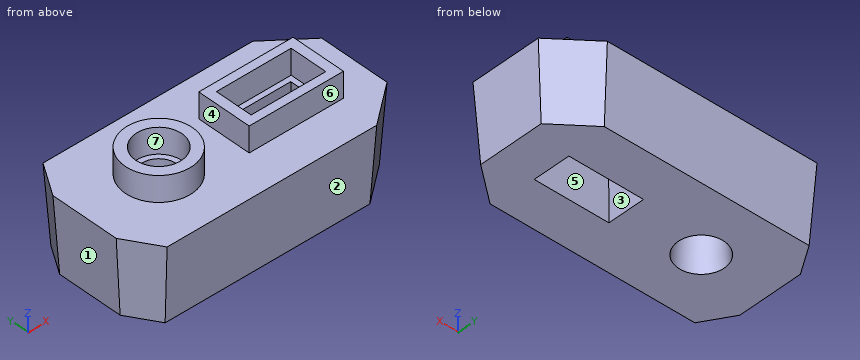
from build123d import *

# Parameters (mm, degrees)
SKETCH1_R           = 12.7
SKETCH1_W           = 41.2
SKETCH1_H           = 20.6
BOSS_EXTRUDE1_DEPTH = 42
BOSS_EXTRUDE1_DRAFT = -4
SKETCH2_R           = 18.5
SKETCH2_R_2         = 12.7
SKETCH2_W           = 52
SKETCH2_H           = 30
SKETCH2_W_2         = 41.2
SKETCH2_H_2         = 20.6
BOSS_EXTRUDE2_DEPTH = 56


with BuildPart() as part:
    # Sketch1 → Boss-Extrude1 (with draft: the straight prism first)
    with BuildSketch(Plane.XY):
        Polygon((-28, 34), (-38, 18), (-38, -18), (-28, -34), (85, -34), (105, -18), (105, 18), (85, 34), align=None)
        Circle(SKETCH1_R, mode=Mode.SUBTRACT)
        with Locations((62, 0)):
            Rectangle(SKETCH1_W, SKETCH1_H, mode=Mode.SUBTRACT)
    extrude(amount=BOSS_EXTRUDE1_DEPTH)
    # Boss-Extrude1: the draft: its side faces are tilted about the plane it starts from
    boss_extrude1_sides = [part.faces().sort_by_distance(p)[0] for p in [
        (-33, 26, 21),
        (-38, 0, 21),
        (-33, -26, 21),
        (28.5, -34, 21),
        (95, -26, 21),
        (105, 0, 21),
        (95, 26, 21),
        (28.5, 34, 21),
        (-12.7, 0, 21),
        (41.4, 0, 21),
        (62, 10.3, 21),
        (82.6, 0, 21),
        (62, -10.3, 21),
    ]]
    draft(boss_extrude1_sides, Plane.XY, BOSS_EXTRUDE1_DRAFT)

    # Sketch2 → Boss-Extrude2 (add)
    # profile 1 of 2: a face of its own
    with BuildSketch(Plane.XY):
        with Locations(Location((0, 0, 0), (0, 0, 180))):
            Circle(SKETCH2_R)
        with Locations(Location((0, 0, 0), (0, 0, 180))):
            Circle(SKETCH2_R_2, mode=Mode.SUBTRACT)
    # profile 2 of 2: a face of its own
    with BuildSketch(Plane.XY):
        with Locations((62, 0)):
            Rectangle(SKETCH2_W, SKETCH2_H)
        with Locations((62, 0)):
            Rectangle(SKETCH2_W_2, SKETCH2_H_2, mode=Mode.SUBTRACT)
    extrude(amount=BOSS_EXTRUDE2_DEPTH)


solid = part.part
Geometry: final body of the model. Coordinates: model frame, mm. Face numbers are marked on the shaded views. A direction names the side the tool comes from. Coordinates: 2 decimals unless noted, no trailing zeros. Loops run counter-clockwise (first coordinate to the right, second up) from the corner with the lowest first, then second, coordinate; pieces in that order, holes last. Notation, with made-up numbers: M 44,39 L 56,39 A18 cw 56,58 Z; hole C 18,-4 d11. An arc over 180 degrees is marked long. One line per item, written item: value. Start each with the question number.
1) Pin query (flat end, axial travel): P1, Ø4, axis at x = 74.5, z = 48.5, coming from the +Y side; P2, Ø16.5, axis at x = 60.5, y = -1.5, coming from the +Z side; P3, Ø7, axis at x = 58, z = 46, coming from the -Y side. Return the tip coordinate at first contact, or that it passes through.
2) Reachability of the marked faces 4, 5, 6 and 7 from +Z, -Z, +X, -X, +Y, -Y: full face, straight path, thin tool, end or side. Return the list, or none.
3) Cut plane A-A (z = 52). Return loops of the section in (x, y), then the cut area to 3 significant figures.
4) Cut plane B-B (x = 66). Return loops of the section in (y, z).
5) Draft query along Y for the marked faces 1, 2 and 3. Return one class per face: released by +Y, released by -Y, zero draft, split by the parting line, or undercut.
6) Cut plane C-C (y = 0). Return loops of the section in (x, z), then the cut area to 3 significant figures.
7) Cut plane D-D (z = 12). Return loops of the section in (x, y).
8) Material intervals for L1, parallel to Y at x = 0, z = 48.5; L2, parallel to Y at x = 52, z = 54; L3, parallel to X at y = -0.5, z = 28, sorted ascending. Write a range as from..to.
Evaluation:
1. P1: y = 15
1. P2: z = 42
1. P3: y = -15
2. face 4: +Z, +Y, -Y
2. face 5: -Z
2. face 6: +Z, +X, -Y
2. face 7: +Z
3. outline: C 0,0 d37; M 36,-15 L 88,-15 L 88,15 L 36,15 Z; hole C 0,0 d25.4; hole M 41.4,-10.3 L 82.6,-10.3 L 82.6,10.3 L 41.4,10.3 Z
3. area: 1,280 mm^2
4. outline: M -36.94,42 L -34,0 L -10.3,0 L -7.36,42 L -10.3,42 L -10.3,56 L -15,56 L -15,42 Z; M 7.36,42 L 10.3,0 L 34,0 L 36.94,42 L 15,42 L 15,56 L 10.3,56 L 10.3,42 Z
5. face 1: zero draft
5. face 2: released by -Y
5. face 3: undercut
6. outline: M -40.94,42 L -38,0 L -12.7,0 L -9.76,42 L -12.7,42 L -12.7,56 L -18.5,56 L -18.5,42 Z; M 9.76,42 L 12.7,0 L 41.4,0 L 44.34,42 L 41.4,42 L 41.4,56 L 36,56 L 36,42 L 18.5,42 L 18.5,56 L 12.7,56 L 12.7,42 Z; M 79.66,42 L 82.6,0 L 105,0 L 107.94,42 L 88,42 L 88,56 L 82.6,56 L 82.6,42 Z
6. area: 3,890 mm^2
7. outline: M -38.84,-18.24 L -28.47,-34.84 L 85.29,-34.84 L 105.84,-18.4 L 105.84,18.4 L 85.29,34.84 L -28.47,34.84 L -38.84,18.24 Z; hole C 0,0 d23.72; hole M 42.24,-9.46 L 81.76,-9.46 L 81.76,9.46 L 42.24,9.46 Z
8. L1: -18.5..-12.7, 12.7..18.5
8. L2: -15..-10.3, 10.3..15
8. L3: -39.96..-10.73, 10.73..43.36, 80.64..106.96
